Check sheet for the modelled part. Datum: model origin and axes. Units: mm. Round coordinates to 2 decimals unless told otherwise and drop trailing zeros. Write each loop counter-clockwise with the first axis right and the second up, starting at its lowest first coordinate (ties: lowest second). Pieces come first, ordered by that corner, then holes.
Item 1: Cross-section at C-C on x = 15.5. Enter the section's corners in (y, z), plus the area to 3 significant figures.
Item 2: Go/stop test with flat-tipped pins: pin 1 Ø8 at (y, z) = (4.5, -51) entering from -X; pin 2 Ø10 at (x, z) = (10, -41) entering from -Y; pin 3 Ø12 at (x, y) = (13.5, -7) entering from -Z. Record where each tip stops, or that it passes through.
Item 3: Material ranges on line 1 (Z direction, x = 3, y = -10); line 2 (X direction, y = -9.5, z = -34.5); line 3 (X direction, y = -4.5, z = 47), recorded low to high.
Item 4: Cross-section at A-A on y = 0. Enter the section's corners in (x, z).
Item 5: Cross-section at B-B on z = 41. Enter the section's corners in (x, y).
from build123d import *

# Parameters (mm, degrees)
SKETCH_1_W               = 50
SKETCH_1_H               = 26
EXTRUDE_1_DEPTH          = 65
SKETCH_7_W               = 20
SKETCH_7_H               = 26
CUT_EXTRUDE_5_DEPTH      = 50
SKETCH_4_R               = 3
EXTRUDE_3_DEPTH          = 40
SKETCH_5_W               = 12.2
SKETCH_5_H               = 8
CUT_EXTRUDE_3_DEPTH      = 4
SKETCH_6_R               = 1
CUT_EXTRUDE_4_DEPTH      = 40
MIRROR_2_COPY_1_SKETCH_W = 20
MIRROR_2_COPY_1_SKETCH_H = 26
MIRROR_2_COPY_1_DEPTH    = 50
MIRROR_2_COPY_2_SKETCH_R = 3
MIRROR_2_COPY_2_DEPTH    = 40
MIRROR_2_COPY_3_SKETCH_W = 12.2
MIRROR_2_COPY_3_SKETCH_H = 8
MIRROR_2_COPY_3_DEPTH    = 4
MIRROR_2_COPY_4_SKETCH_R = 1
MIRROR_2_COPY_4_DEPTH    = 40
CUT_EXTRUDE_7_DEPTH      = 71.89816586
CUT_EXTRUDE_7_DEPTH_BACK = 71.89816586
CUT_EXTRUDE_8_REACH      = 86.862


with BuildPart() as part:
    # Эскиз1 → Бобышка-Вытянуть1 (new, symmetric)
    with BuildSketch(Plane.XY):
        with Locations((0, -0.287208972)):
            Rectangle(SKETCH_1_W, SKETCH_1_H)
    extrude(amount=EXTRUDE_1_DEPTH, both=True)

    # Эскиз7 → Вырез-Вытянуть5 (cut)
    with BuildSketch(Plane.XY.offset(65)):
        with Locations((-15, -0.287208972)):
            Rectangle(SKETCH_7_W, SKETCH_7_H)
    cut_extrude_5 = extrude(amount=-CUT_EXTRUDE_5_DEPTH, mode=Mode.SUBTRACT)

    # Эскиз4 → Бобышка-Вытянуть3 (add)
    with BuildSketch(Plane.XY.offset(65)):
        with Locations((-5, -10.287208972)):
            Circle(SKETCH_4_R)
    extrude_3 = extrude(amount=-EXTRUDE_3_DEPTH)

    # Эскиз5 → Вырез-Вытянуть3 (cut, symmetric)
    with BuildSketch(Plane.ZY.offset(5)):
        with Locations((44.95, -9.287208972)):
            Rectangle(SKETCH_5_W, SKETCH_5_H)
    cut_extrude_3 = extrude(amount=CUT_EXTRUDE_3_DEPTH, both=True, mode=Mode.SUBTRACT)

    # Эскиз6 → Вырез-Вытянуть4 (cut)
    with BuildSketch(Plane.XY.offset(65)):
        with Locations((-5, -10.287208972)):
            Circle(SKETCH_6_R)
    cut_extrude_4 = extrude(amount=-CUT_EXTRUDE_4_DEPTH, mode=Mode.SUBTRACT)

    # Зеркальное отражение1: Вырез-Вытянуть5, Бобышка-Вытянуть3, Вырез-Вытянуть3, Вырез-Вытянуть4 across plane
    add(cut_extrude_5.mirror(Plane.XY), mode=Mode.SUBTRACT)
    add(extrude_3.mirror(Plane.XY))
    add(cut_extrude_3.mirror(Plane.XY), mode=Mode.SUBTRACT)
    add(cut_extrude_4.mirror(Plane.XY), mode=Mode.SUBTRACT)

    # Зеркальное отражение2: Вырез-Вытянуть5, Бобышка-Вытянуть3, Вырез-Вытянуть3, Вырез-Вытянуть4 across plane
    add(cut_extrude_5.mirror(Plane(origin=(0, 0, 0), x_dir=(0, 0, 1), z_dir=(1, 0, 0))), mode=Mode.SUBTRACT)
    add(extrude_3.mirror(Plane(origin=(0, 0, 0), x_dir=(0, 0, 1), z_dir=(1, 0, 0))))
    add(cut_extrude_3.mirror(Plane(origin=(0, 0, 0), x_dir=(0, 0, 1), z_dir=(1, 0, 0))), mode=Mode.SUBTRACT)
    add(cut_extrude_4.mirror(Plane(origin=(0, 0, 0), x_dir=(0, 0, 1), z_dir=(1, 0, 0))), mode=Mode.SUBTRACT)

    # Зеркальное отражение2 copy 1 sketch → Зеркальное отражение2 copy 1 (cut)
    with BuildSketch(Plane(origin=(0, 0, -65), x_dir=(-1, 0, 0), z_dir=(0, 0, -1))):
        with Locations((-15, -0.287208972)):
            Rectangle(MIRROR_2_COPY_1_SKETCH_W, MIRROR_2_COPY_1_SKETCH_H)
    extrude(amount=-MIRROR_2_COPY_1_DEPTH, mode=Mode.SUBTRACT)

    # Зеркальное отражение2 copy 2 sketch → Зеркальное отражение2 copy 2 (add)
    with BuildSketch(Plane(origin=(0, 0, -65), x_dir=(-1, 0, 0), z_dir=(0, 0, -1))):
        with Locations((-5, -10.287208972)):
            Circle(MIRROR_2_COPY_2_SKETCH_R)
    extrude(amount=-MIRROR_2_COPY_2_DEPTH)

    # Зеркальное отражение2 copy 3 sketch → Зеркальное отражение2 copy 3 (cut, symmetric)
    with BuildSketch(Plane(origin=(5, 0, 0), x_dir=(0, 0, -1), z_dir=(1, 0, 0))):
        with Locations((44.95, -9.287208972)):
            Rectangle(MIRROR_2_COPY_3_SKETCH_W, MIRROR_2_COPY_3_SKETCH_H)
    extrude(amount=MIRROR_2_COPY_3_DEPTH, both=True, mode=Mode.SUBTRACT)

    # Зеркальное отражение2 copy 4 sketch → Зеркальное отражение2 copy 4 (cut)
    with BuildSketch(Plane(origin=(0, 0, -65), x_dir=(-1, 0, 0), z_dir=(0, 0, -1))):
        with Locations((-5, -10.287208972)):
            Circle(MIRROR_2_COPY_4_SKETCH_R)
    extrude(amount=-MIRROR_2_COPY_4_DEPTH, mode=Mode.SUBTRACT)

    # Эскиз9 → Вырез-Вытянуть7 (cut, two sides: drawn at the far end of the back side and taken through both)
    with BuildSketch(Plane.XY.offset(-CUT_EXTRUDE_7_DEPTH_BACK)):
        with BuildLine():
            Line((0, -9.287208972), (0, 8.712791028))
            Line((0, 8.712791028), (-0.101020514, 8.712791028))
            ThreePointArc((-0.101020514, 8.712791028), (-0.775255129, 7.038556414), (-2, 5.712791028))
            Line((-2, 5.712791028), (-2, -6.287208972))
            ThreePointArc((-2, -6.287208972), (-0.775255129, -7.612974358), (-0.101020514, -9.287208972))
            Line((-0.101020514, -9.287208972), (0, -9.287208972))
        make_face()
        with BuildLine():
            Line((0.101020514, 8.712791028), (0, 8.712791028))
            Line((0, 8.712791028), (0, -9.287208972))
            Line((0, -9.287208972), (0.101020514, -9.287208972))
            ThreePointArc((0.101020514, -9.287208972), (0.775255129, -7.612974358), (2, -6.287208972))
            Line((2, -6.287208972), (2, 5.712791028))
            ThreePointArc((2, 5.712791028), (0.775255129, 7.038556414), (0.101020514, 8.712791028))
        make_face()
    extrude(amount=CUT_EXTRUDE_7_DEPTH + CUT_EXTRUDE_7_DEPTH_BACK, mode=Mode.SUBTRACT)

    # Эскиз10 → Вырез-Вытянуть8 (cut, up to next)
    with BuildSketch(Plane.XY.offset(15), mode=Mode.PRIVATE) as cut_extrude_8_sk1:
        Polygon((-20, -13.287208972), (-25, -8.287208972), (-25, -13.287208972), align=None)
    cut_extrude_8_tool1 = extrude(cut_extrude_8_sk1.sketch, amount=-CUT_EXTRUDE_8_REACH, mode=Mode.PRIVATE) & part.part
    # Эскиз10 → Вырез-Вытянуть8 (cut, up to next)
    with BuildSketch(Plane.XY.offset(15), mode=Mode.PRIVATE) as cut_extrude_8_sk2:
        Polygon((20, -13.287208972), (25, -13.287208972), (25, -8.287208972), align=None)
    cut_extrude_8_tool2 = extrude(cut_extrude_8_sk2.sketch, amount=-CUT_EXTRUDE_8_REACH, mode=Mode.PRIVATE) & part.part
    add(cut_extrude_8_tool1.solids().sort_by_distance((-23.333333, -11.620542, 15))[0], mode=Mode.SUBTRACT)
    add(cut_extrude_8_tool2.solids().sort_by_distance((23.333333, -11.620542, 15))[0], mode=Mode.SUBTRACT)


solid = part.part
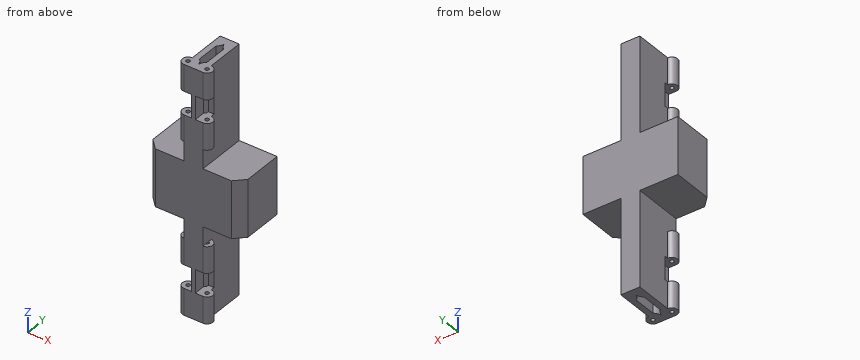
Response values:
1. outline: (-13.29, -15) - (12.71, -15) - (12.71, 15) - (-13.29, 15) - close
1. area: 780 mm2
2. pin 1: stops at x = -5
2. pin 2: stops at y = -13.25
2. pin 3: stops at z = -15
3. line 1: z = -65 to -51.05, -38.85 to 38.85, 51.05 to 65
3. line 2: x = -7.89 to -5.62, -4.38 to 4.38, 5.62 to 7.89
3. line 3: x = -5 to -2, 2 to 5
4. outline: (-25, -15) - (-5, -15) - (-5, -65) - (-2, -65) - (-2, 65) - (-5, 65) - (-5, 15) - (-25, 15) - close; (2, -65) - (5, -65) - (5, -15) - (25, -15) - (25, 15) - (5, 15) - (5, 65) - (2, 65) - close
5. outline: (-5, -5.29) - (-2, -5.29) - (-2, 5.71) arc R5 ccw to (-0.1, 8.71) - (0.1, 8.71) arc R5 ccw to (2, 5.71) - (2, -5.29) - (5, -5.29) - (5, 12.71) - (-5, 12.71) - close; (-1, -13.29) - (1, -13.29) - (1, -7.29) arc R5 ccw to (0.1, -9.29) - (-0.1, -9.29) arc R5 ccw to (-1, -7.29) - close
